```python
from build123d import *

# Parameters (mm, degrees)
SKETCH_R        = 3.55854
SKETCH_R_2      = 3.1877
PAD_DEPTH       = 5.5245
SKETCH001_R     = 16.81734
PAD001_DEPTH    = 6.1214
SKETCH002_R     = 14.78534
POCKET_DEPTH    = 2.4765
SKETCH003_R     = 6.9723
PAD002_DEPTH    = 3.1877
SKETCH004_R     = 3.1877
POCKET001_DEPTH = 12.3581


with BuildPart() as part:
    # Sketch → Pad (new body)
    with BuildSketch(Plane.XY):
        with BuildLine():
            ThreePointArc((-15.148609, -9.525), (0, -17.8943), (15.148609, -9.525))
            Line((29.8196, -3.81), (15.148609, -9.525))
            Line((29.8196, 3.81), (29.8196, -3.81))
            Line((29.8196, 3.81), (15.148609, 9.525))
            ThreePointArc((15.148609, 9.525), (0, 17.8943), (-15.148609, 9.525))
            Line((-29.8196, 3.81), (-15.148609, 9.525))
            Line((-29.8196, 3.81), (-29.8196, -3.81))
            Line((-29.8196, -3.81), (-15.148609, -9.525))
        make_face()
        with Locations((22.32025, 0)):
            Circle(SKETCH_R, mode=Mode.SUBTRACT)
        with Locations((-22.32025, 0)):
            Circle(SKETCH_R, mode=Mode.SUBTRACT)
        Circle(SKETCH_R_2, mode=Mode.SUBTRACT)
    extrude(amount=PAD_DEPTH)

    # Sketch001 → Pad001 (new body)
    with BuildSketch(Plane.XY.offset(5.5245)):
        Circle(SKETCH001_R)
    extrude(amount=PAD001_DEPTH)

    # Sketch002 → Pocket (cut)
    with BuildSketch(Plane.XY.offset(11.6459)):
        Circle(SKETCH002_R)
    extrude(amount=-POCKET_DEPTH, mode=Mode.SUBTRACT)

    # Sketch003 → Pad002 (new body)
    with BuildSketch(Plane.XY.offset(9.1694)):
        Circle(SKETCH003_R)
    extrude(amount=PAD002_DEPTH)

    # Sketch004 → Pocket001 (cut, through all)
    with BuildSketch(Plane.XY.offset(12.3571)):
        Circle(SKETCH004_R)
    extrude(amount=-POCKET001_DEPTH, mode=Mode.SUBTRACT)


solid = part.part
```
Work out the finished part from the listing and answer in its coordinate system (mm). A direction names the side the tool comes from. Coordinates: 2 decimals unless noted, no trailing zeros. Loops run counter-clockwise (first coordinate to the right, second up) from the corner with the lowest first, then second, coordinate; pieces in that order, holes last.
1) Section B-B (z = 1.25) is taken. Give the vertices of the cut face in (x, y) (3 decimals), plus the area to 3 significant figures.
Results:
outline: (-29.82, -3.81) - (-15.149, -9.525) arc R17.894 ccw to (15.149, -9.525) - (29.82, -3.81) - (29.82, 3.81) - (15.149, 9.525) arc R17.894 ccw to (-15.149, 9.525) - (-29.82, 3.81) - close; hole circle Ø7.117 at (-22.32, 0); hole circle Ø6.375 at (0, 0); hole circle Ø7.117 at (22.32, 0)
area: 1,210 mm2
2) For faces 4 (the flat face through (29.82, 0, 3)), 5 (the cylindrical face through (-3.646, -16.417, 8.542)), determine the directions among +Z, -Z, +X, -X, +Y, -Y from which every point of the face is accessible in a straight line to the end or side of a thin tool.
Results:
face 4: +Z, -Z, +X, +Y, -Y
face 5: +Z
3) Flat-ended cylindrical pins translate along their axes: pin 1 (3 mm diameter, centred on x = -4, z = 6, fed in from -Y); pin 2 (8 mm diameter, centred on x = -22.32, y = 0, fed in from -Z); pin 3 (1.5 mm diameter, centred on y = 11.5, z = 3, fed in from -X); pin 4 (6 mm diameter, centred on x = -17.5, y = -3, fed in from +Z). Find the tip coordinate at first contact, or state that the pin passes through.
Results:
pin 1: stops at y = -17.71
pin 2: stops at z = 0
pin 3: stops at x = -14.31
pin 4: stops at z = 11.65
4) Section D-D (z = 10) is taken. Give the vertices of the cut face in (x, y).
Results:
outline: circle Ø33.63 at (0, 0); circle Ø13.94 at (0, 0); hole circle Ø29.57 at (0, 0); hole circle Ø6.38 at (0, 0)
5) Consider probe 1 along Y at (x, z) = (0, 10.1); probe 2 along Z at (x, y) = (-6, 9); probe 3 along Z at (x, y) = (-15, -9). Determine where each line is inside the solid, lowest interval first.
Results:
probe 1: y = -16.82 to -14.79, -6.97 to -3.19, 3.19 to 6.97, 14.79 to 16.82
probe 2: z = 0 to 9.17
probe 3: z = 0 to 5.52
6) Section A-A (y = 0) is taken. Give the vertices of the cut face in (x, z), plus the area to 3 significant figures.
Results:
outline: (-29.82, 0) - (-25.88, 0) - (-25.88, 5.52) - (-29.82, 5.52) - close; (-18.76, 0) - (-3.19, 0) - (-3.19, 12.36) - (-6.97, 12.36) - (-6.97, 9.17) - (-14.79, 9.17) - (-14.79, 11.65) - (-16.82, 11.65) - (-16.82, 5.52) - (-18.76, 5.52) - close; (3.19, 0) - (18.76, 0) - (18.76, 5.52) - (16.82, 5.52) - (16.82, 11.65) - (14.79, 11.65) - (14.79, 9.17) - (6.97, 9.17) - (6.97, 12.36) - (3.19, 12.36) - close; (25.88, 0) - (29.82, 0) - (29.82, 5.52) - (25.88, 5.52) - close
area: 349 mm2
7) Section C-C (x = 0) is taken. Give the vertices of the cut face in (y, z).
Results:
outline: (-17.89, 0) - (-3.19, 0) - (-3.19, 12.36) - (-6.97, 12.36) - (-6.97, 9.17) - (-14.79, 9.17) - (-14.79, 11.65) - (-16.82, 11.65) - (-16.82, 5.52) - (-17.89, 5.52) - close; (3.19, 0) - (17.89, 0) - (17.89, 5.52) - (16.82, 5.52) - (16.82, 11.65) - (14.79, 11.65) - (14.79, 9.17) - (6.97, 9.17) - (6.97, 12.36) - (3.19, 12.36) - close
8) For a pull along Y with two mould halves and no side action, classify faces 1 (the flat face through (0, -4, 0)), 2 (the flat face through (-22.587, -6.627, 2.724)), 3 (the cylindrical face through (1.47, -2.83, 6.09)) as +Y half, -Y half, draft (parallel to the pull), parting line (faces both ways), or undercut.
Results:
face 1: draft
face 2: -Y half
face 3: undercut
